Geometry: final body of the model. Coordinates: model frame, mm. A direction names the side the tool comes from. Coordinates: 2 decimals unless noted, no trailing zeros. Order: outer loops, then holes, each group sorted by start corner. A loop starts at its lowest first (then second) coordinate and runs counter-clockwise, first axis right, second up. Notation, with made-up numbers: (-18, 15.25) -> (-6, 15.25) arc R26 ccw to (-6, 30.25) -> close; hole circle Ø1 at (13.25, -19). An arc over 180 degrees is marked (long way). Answer in a Markdown table with one row per item. Add a question column.
1) Pull-direction query (Z, two-part tool) for faces 3 (the face through (-12, -76.2, -27)), 4 (the face through (31.39, -37.57, 9.89)), 5 (the face through (21.53, -41.76, -19.74)); classes: +Z half, -Z half, draft (parallel to the pull), parting line (faces both ways), or undercut.
2) Ray query, line 1 (Z direction, x = 0, y = -42); line 2 (Y direction, x = -17, z = -19); line 3 (X direction, y = -15, z = 23.5). Return the intervals inside material, ascending. Write a range as from..to.
3) Contact query for flat-ended pins moving along their axis: P1, Ø3, axis at x = 22, z = -8.5, coming from the -Y side; P2, Ø4, axis at y = -53.5, z = -20.5, coming from the -X side; P3, Ø5, axis at y = -57, z = -21.5, coming from the +X side. Output: stop coordinate, or through.
4) Set-up query: faces 1 (the face through (0, -6.35, 0)), 2 (the face through (0, 0, 0)). Return all of +Z, -Z, +X, -X, +Y, -Y with unobstructed straight access to the full face (end or side cutting, diameter ignored); none if empty.
5) Section query B-B on x = 0. Return the cut outline in (y, z), then the cut area to 3 significant figures.
6) Section query C-C on z = -7. Return the cut outline in (x, y).
7) Section query A-A on y = -55. Return the cut outline in (x, z), then the cut area to 3 significant figures.
```python
from build123d import *

# Parameters (mm, degrees)
F0_R     = 32.909894
F2_DEPTH = 76.2
F3_D     = 58.42
F4_R     = 30.278142
F5_DEPTH = 6.35


with BuildPart() as f2:
    # F0 (on Front) → F2 (new body)
    with BuildSketch(Plane.XZ):
        Circle(F0_R)
    extrude(amount=F2_DEPTH)

    # F3 (through all)
    with Locations(Plane(origin=(0, 0, 0), x_dir=(1, 0, 0), z_dir=(0, 1, 0))):
        with Locations((0, 0)):
            Hole(F3_D / 2)

    # F4 (on Front) → F5 (join)
    with BuildSketch(Plane.XZ):
        Circle(F4_R)
    extrude(amount=F5_DEPTH)


solid = f2.part
```
Result:
| question | item | result |
|---|---|---|
| 1 | face 3 | draft |
| 1 | face 4 | parting line |
| 1 | face 5 | undercut |
| 2 | line 1 | -32.91..-29.21, 29.21..32.91 |
| 2 | line 2 | -6.35..0 |
| 2 | line 3 | -23.04..-17.35, 17.35..23.04 |
| 3 | P1 | y = -6.35 |
| 3 | P2 | x = -27.22 |
| 3 | P3 | x = 26.87 |
| 4 | face 1 | -Y |
| 4 | face 2 | +Z, -Z, +X, -X, +Y |
| 5 | outline | (-76.2, -32.91) -> (0, -32.91) -> (0, 32.91) -> (-76.2, 32.91) -> (-76.2, 29.21) -> (-6.35, 29.21) -> (-6.35, -29.21) -> (-76.2, -29.21) -> close |
| 5 | area | 935 mm2 |
| 6 | outline | (-32.16, -76.2) -> (-28.36, -76.2) -> (-28.36, -6.35) -> (28.36, -6.35) -> (28.36, -76.2) -> (32.16, -76.2) -> (32.16, 0) -> (-32.16, 0) -> close |
| 7 | outline | circle Ø65.82 at (0, 0); hole circle Ø58.42 at (0, 0) |
| 7 | area | 722 mm2 |
